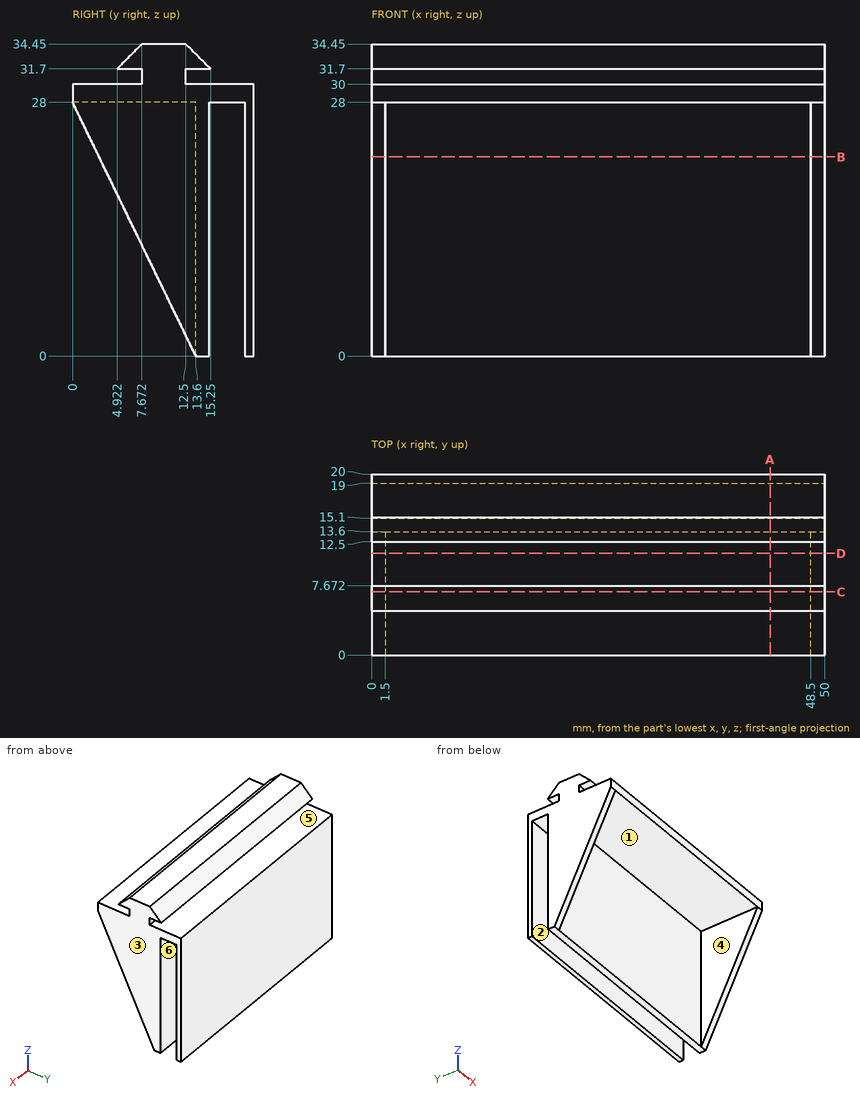
Geometry check sheet. Reference: drawing and pictorial views, mm from the part's lowest x, y, z. A direction names the side the tool comes from. Give positions to 0.01 mm unless a question says otherwise; leave off trailing zeros. Order: outer loops, then holes, each group sorted by start corner. A loop starts at its lowest first (then second) coordinate and runs counter-clockwise, first axis right, second up. Notation, with made-up numbers: (-17, 5) -> (-7, 5) arc R16 cw to (-7, 13) -> close; hole circle Ø11 at (70.25, 86). An arc over 180 degrees is marked (long way). Use CSV: the item, a comma, the result in double quotes. Start each with the question number.
1) Sectioned sample at A-A, the plane x = 44. Record the boundary of the cut face in (y, z), plus the area to 3 significant figures.
2) Go/stop test with flat-tipped pins: P1, Ø11, axis at x = 27, y = 3.5, coming from the -Z side; P2, Ø1.9, axis at x = 23.5, z = 31, coming from the +Y side; P3, Ø2.5, axis at x = 21.5, y = 5, coming from the +Z side. Record where each tip stops, or that it passes through.
3) Mould release check, pull along X, two halves, no side actions. Record for the marked faces 1, 2 and 3: released by +X, released by -X, zero draft, split by the parting line, or undercut.
4) Sectioned sample at B-B, the plane z = 22. Record the boundary of the cut face in (x, y).
5) Material ranges on line 1 (Y direction, x = 25, z = 21); line 2 (X direction, y = 9.5, z = 13); line 3 (Z direction, x = 19.5, y = 3.75), recorded low to high. Write a range as from..to.
6) Sectioned sample at C-C, the plane y = 7. Record the boundary of the cut face in (x, z), plus the area to 3 significant figures.
7) Set-up check for the marked faces 4, 5 and 6: record each of +Z, -Z, +X, -X, +Y, -Y from which the full face is reachable in a straight line by a thin tool's end or side.
8) Sectioned sample at D-D, the plane y = 11.25. Record the boundary of the cut face in (x, z), plus the area to 3 significant figures.
Recorded:
1,outline,"(0, 28) -> (13.6, 28) -> (13.6, 0) -> (15.1, 0) -> (15.1, 28) -> (19, 28) -> (19, 0) -> (20, 0) -> (20, 30) -> (12.5, 30) -> (12.5, 31.7) -> (15.25, 31.7) -> (12.5, 34.45) -> (7.67, 34.45) -> (4.92, 31.7) -> (7.67, 31.7) -> (7.67, 30) -> (0, 30) -> close"
1,area,"139 mm2"
2,P1,"z = 28"
2,P2,"y = 15.25"
2,P3,"z = 33.03"
3,face 1,"undercut"
3,face 2,"zero draft"
3,face 3,"released by +X"
4,outline,"(0, 2.91) -> (1.5, 2.91) -> (1.5, 13.6) -> (48.5, 13.6) -> (48.5, 2.91) -> (50, 2.91) -> (50, 15.1) -> (0, 15.1) -> close; (0, 19) -> (50, 19) -> (50, 20) -> (0, 20) -> close"
5,line 1,"13.6..15.1, 19..20"
5,line 2,"0..1.5, 48.5..50"
5,line 3,"28..30"
6,outline,"(0, 13.59) -> (1.5, 13.59) -> (1.5, 28) -> (48.5, 28) -> (48.5, 13.59) -> (50, 13.59) -> (50, 30) -> (0, 30) -> close; (0, 31.7) -> (50, 31.7) -> (50, 33.78) -> (0, 33.78) -> close"
6,area,"247 mm2"
7,face 4,"-Z, -Y"
7,face 5,"+X, -X, +Y"
7,face 6,"-Z, +X, -X"
8,outline,"(0, 4.84) -> (1.5, 4.84) -> (1.5, 28) -> (48.5, 28) -> (48.5, 4.84) -> (50, 4.84) -> (50, 34.45) -> (0, 34.45) -> close"
8,area,"392 mm2"
